The drawing under review shows one solid part. Ordinate dimensions are in mm from its lowest x, y, z. A direction names the side the tool comes from. Round coordinates to 2 decimals unless told otherwise and drop trailing zeros. Order: outer loops, then holes, each group sorted by start corner. A loop starts at its lowest first (then second) coordinate and runs counter-clockwise, first axis right, second up. Notation, with made-up numbers: M 8,34.5 L 30,34.5 A12 cw 30,51.5 Z; hole C 68,87 d5. An arc over 180 degrees is marked long. Answer as a JSON object with one key per item and string values. Group by question number.
1. Mouldability with a two-part tool opening along Z and no side actions: class the marked faces 1, 2 and 3 as released by +Z, released by -Z, zero draft, split by the parting line, or undercut.
2. Add section A-A on x = 5. State the section outline as (y, z) points.
3. Machinability: for the marked faces 4, 5 and 6, which of the approach directions +Z, -Z, +X, -X, +Y, -Y give a long, thin tool a straight path to every point of the face, cutting with its end or side? Answer none if there is none.
4. To check wall thickness, follow probe 1 along Y at (x, z) = (5, 3.5); probe 2 along Z at (x, y) = (7, 15.75) (1 decimal); probe 3 along Z at (x, y) = (5.25, 9) (1 decimal). State the ranges of each line that lie inside material, in increasing order. Write a range as [from, to].
5. Clearance check with flat-ended pins moving along their axes: P1, Ø4.5, axis at x = 10, y = 10.5, coming from the -Z side; P2, Ø10, axis at y = 12, z = 2.5, coming from the -X side; P3, Ø1, axis at y = 14, z = 11, coming from the -X side; P4, Ø4, axis at x = 13, z = 4, coming from the +Y side. State where each tip first meets the part, or that it passes through.
6. Add section C-C on y = 3. State the section outline as (x, z) points.
7. Add section D-D on x = 1.5. State the section outline as (y, z) points.
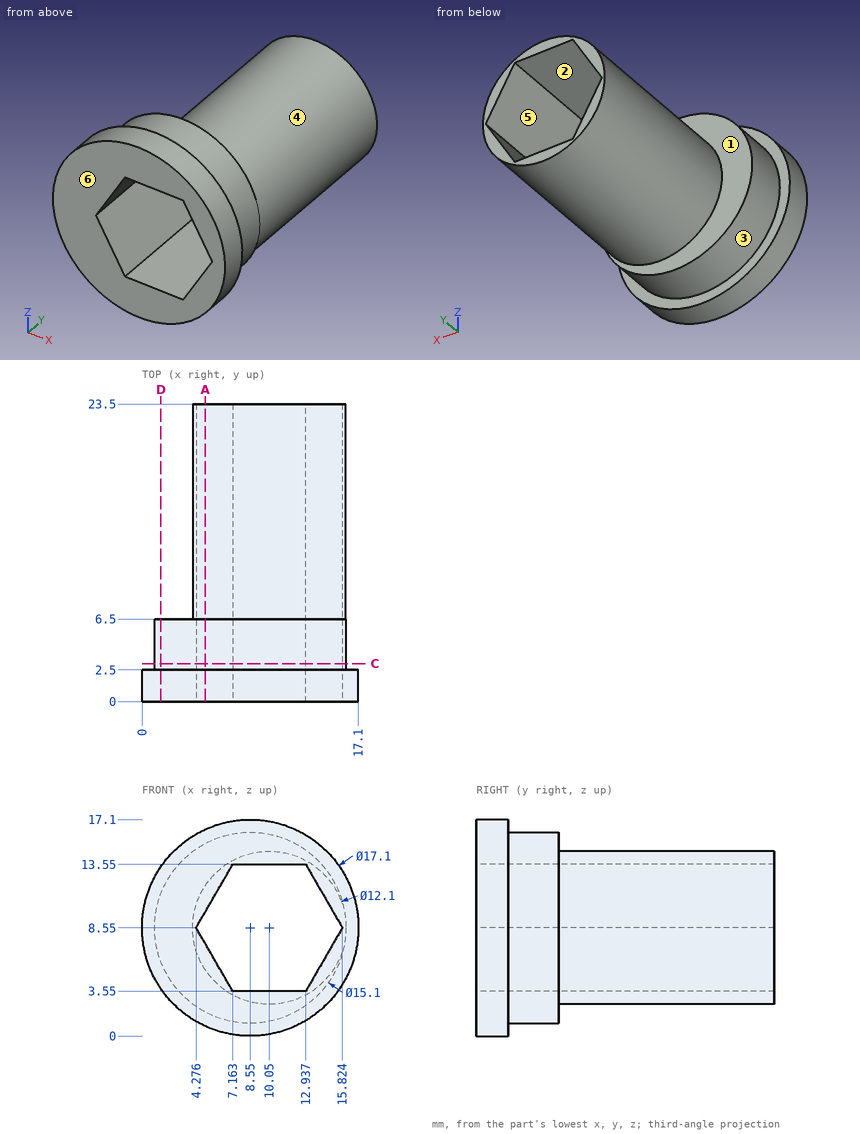
Recorded:
{
 "1": {"face 1": "zero draft", "face 2": "undercut", "face 3": "split by the parting line"},
 "2": {"outline": "M 0,0.77 L 2.5,0.77 L 2.5,1.89 L 6.5,1.89 L 6.5,5.22 L 23.5,5.22 L 23.5,7.3 L 0,7.3 Z; M 0,9.8 L 23.5,9.8 L 23.5,11.88 L 6.5,11.88 L 6.5,15.21 L 2.5,15.21 L 2.5,16.33 L 0,16.33 Z"},
 "3": {"face 4": "+Y", "face 5": "+Y, -Y", "face 6": "+Z, -Z, +X, -X, -Y"},
 "4": {"probe 1": "y = [0, 6.5]", "probe 2": "z = [3.3, 3.8], [13.3, 13.8]", "probe 3": "z = [4.9, 6.9], [10.2, 12.2]"},
 "5": {"P1": "stops at z = 2.5", "P2": "stops at x = 4.09", "P3": "stops at x = 4.32", "P4": "stops at y = 23.5"},
 "6": {"outline": "C 8.55,8.55 d15.1; hole M 4.28,8.55 L 7.16,3.55 L 12.94,3.55 L 15.82,8.55 L 12.94,13.55 L 7.16,13.55 Z"},
 "7": {"outline": "M 0,3.71 L 2.5,3.71 L 2.5,5.85 L 6.5,5.85 L 6.5,11.25 L 2.5,11.25 L 2.5,13.39 L 0,13.39 Z"}
}
